```python
from build123d import *

# Parameters (mm, degrees)
BASEPLATE_W                   = 200
BASEPLATE_H                   = 200
BOSS_EXTRUDE1_DEPTH           = 3
FILLET1_R                     = 3
F_5_32_DOWEL_HOLE_D           = 3.96875
F_5_32_DOWEL_HOLE_CSINK_D     = 5.23875
F_5_32_DOWEL_HOLE_CSINK_ANGLE = 100


with BuildPart() as part:
    # Baseplate → Boss-Extrude1 (new body)
    with BuildSketch(Plane.XY):
        Rectangle(BASEPLATE_W, BASEPLATE_H)
    extrude(amount=BOSS_EXTRUDE1_DEPTH)

    # Fillet1
    fillet1_edges = [part.edges().sort_by_distance(p)[0] for p in [
        (100, -100, 1.5),
        (-100, -100, 1.5),
        (-100, 100, 1.5),
        (100, 100, 1.5),
    ]]
    fillet(fillet1_edges, radius=FILLET1_R)

    # Sketch8 → 1/4 Inch Bolt Hole (revolve, cut)
    with BuildSketch(Plane.YZ):
        Polygon((0, 0), (0, 3), (3.175, 3), (3.175, 0.635), (3.81, 0), align=None)
    revolve(axis=Axis((0, 0, -6.35), (0, 0, 1)), mode=Mode.SUBTRACT)

    # 5/32 Dowel Hole (through all)
    with Locations(Plane(origin=(0, 0, 0), x_dir=(-1, 0, 0), z_dir=(0, 0, -1))):
        with Locations((-44.5, 0), (44.45, 0)):
            CounterSinkHole(F_5_32_DOWEL_HOLE_D / 2, F_5_32_DOWEL_HOLE_CSINK_D / 2, counter_sink_angle=F_5_32_DOWEL_HOLE_CSINK_ANGLE)


solid = part.part
```
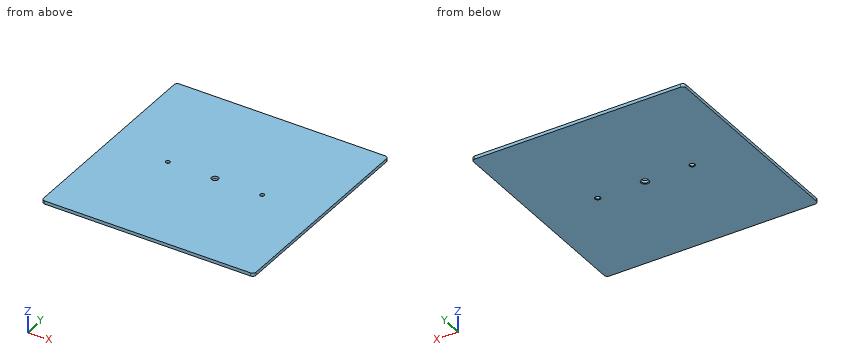
Source: CAD feature listing. Evaluate the final solid. Frame: model axes, mm. Give positions to 0.01 mm unless a question says otherwise; leave off trailing zeros. Loops run counter-clockwise (first coordinate to the right, second up) from the corner with the lowest first, then second, coordinate; pieces in that order, holes last. Notation, with made-up numbers: (28.25, 66) -> (61.25, 66) arc R29 cw to (61.25, 90) -> close; hole circle Ø4 at (-1.75, 62). An arc over 180 degrees is marked (long way). Put each result on its own line as item: value. Start each with the question number.
1) Material intervals for probe 1 along X at (y, z) = (0, 1.05) (3 decimals); probe 2 along Y at (x, z) = (-44.45, 1.35); probe 3 along X at (y, z) = (-0.5, 0.75), sorted ascending.
2) Contact query for flat-ended pins moving along their axis: P1, Ø3.5, axis at x = 44.5, y = 0, coming from the -Z side; P2, Ø5, axis at x = -44.45, y = 0, coming from the -Z side. Output: stop coordinate, or through.
3) Cut plane A-A (x = 0). Return loops of the section in (y, z) (3 decimals), then the cut area to 3 significant figures.
Results are:
1. probe 1: x = -100 to -46.434, -42.466 to -3.175, 3.175 to 42.516, 46.484 to 100
1. probe 2: y = -100 to -1.98, 1.98 to 100
1. probe 3: x = -100 to -46.37, -42.53 to -3.14, 3.14 to 42.58, 46.42 to 100
2. P1: passes through
2. P2: stops at z = 0.1
3. outline: (-100, 0) -> (-3.81, 0) -> (-3.175, 0.635) -> (-3.175, 3) -> (-100, 3) -> close; (3.175, 0.635) -> (3.81, 0) -> (100, 0) -> (100, 3) -> (3.175, 3) -> close
3. area: 581 mm2
